Solid Edge part; units mm, degrees
sketch "Sketch1" plane through (0, 0, 0) normal (0, -1, 0) x (1, 0, 0)
  line L0 (270, 170) -> (-270, 170)
  line L1 (-270, 170) -> (-270, -170)
  line L2 (-270, -170) -> (270, -170)
  line L3 (270, -170) -> (270, 170)
  line L4 (330, 230) -> (-330, 230)
  line L5 (-330, 230) -> (-330, -230)
  line L6 (-330, -230) -> (330, -230)
  line L7 (330, -230) -> (330, 230)
extrude "Protrusion1" add sketch "Sketch1" against normal blind 60
sketch "Sketch2" plane through (0, 60, 0) normal (0, 1, 0) x (1, 0, 0)
  line L0 (269.9973, 170.0076) -> (329.9407, 170.0076)
  line L1 (329.9407, 170.0076) -> (329.9407, 229.951)
  line L2 (329.9407, 229.951) -> (269.9973, 229.951)
  line L3 (269.9973, 229.951) -> (269.9973, 170.0076)
extrude "ExtrudedProtrusion_2" add sketch "Sketch2" along normal blind 180
sketch "Sketch3" plane through (329.9407, 150, -199.9793) normal (1, 0, 0) x (0, 0, 1)
  line L0 (-29.9717, -63.4202) -> (29.9717, -63.4202)
  line L1 (29.9717, -63.4202) -> (30.0593, -72.2902)
  line L2 (30.0593, -90.0301) -> (30.0593, -72.2902)
  line L3 (-30.0593, -90.0301) -> (30.0593, -90.0301)
  line L4 (-30.0593, -72.2902) -> (-30.0593, -90.0301)
  line L5 (-30.0593, -72.2902) -> (-29.9717, -63.4202)
extrude "ExtrudedProtrusion_3" add sketch "Sketch3" along normal blind 60
mirror "Mirror1" about plane through (0, 0, 0) normal (-1, 0, 0) of "ExtrudedProtrusion_2", "ExtrudedProtrusion_3"
mirror "Mirror2" about plane through (0, 0, 0) normal (0, 0, 1) of "ExtrudedProtrusion_2", "ExtrudedProtrusion_3"
mirror "Mirror3" about plane through (0, 0, 0) normal (0, 0, 1) of "Mirror1"
sketch "Sketch4" plane through (0, 0, 0) normal (0, -1, 0) x (1, 0, 0)
  circle A0 centre (-300, 152.3787) radius 20
  circle A1 centre (-300, 106.6771) radius 20
  circle A2 centre (-300, 52.3163) radius 20
  circle A3 centre (-300, 0) radius 20
extrude "ExtrudedCutout_8" cut sketch "Sketch4" against normal blind 60
mirror "Mirror4" about plane through (0, 0, 0) normal (-1, 0, 0) of "ExtrudedCutout_8"
mirror "Mirror5" about plane through (0, 0, 0) normal (0, 0, -1) of "ExtrudedCutout_8", "Mirror4"
Input: part model. Units: mm. Frame: model coordinates. A direction names the side the tool comes from. Coordinates: 2 decimals unless noted, no trailing zeros. Write each loop counter-clockwise with the first axis right and the second up, starting at its lowest first coordinate (ties: lowest second). Pieces come first, ordered by that corner, then holes. Notation, with made-up numbers: M 50.5,-9 L 69.5,-9 A21 cw 69.5,-3 Z; hole C -12,17 d6. An arc over 180 degrees is marked long. Use one line per item in the form item = value.
Q1. Material intervals for probe 1 along X at (y, z) = (22, -52); probe 2 along X at (y, z) = (17.5, 22); probe 3 along X at (y, z) = (208.5, -192), sorted ascending. Write a range as from..to.
Answer below:
probe_1 = -330..-320, -280..-270, 270..280, 320..330
probe_2 = -330..-270, 270..330
probe_3 = -329.94..-270, 270..329.94
Q2. Section B-B (z = 0). Return loops of the section in (x, y), plus the area to 3 significant figures.
Answer below:
outline = M -330,0 L -320,0 L -320,60 L -330,60 Z; M -280,0 L -270,0 L -270,60 L -280,60 Z; M 270,0 L 280,0 L 280,60 L 270,60 Z; M 320,0 L 330,0 L 330,60 L 320,60 Z
area = 2,400 mm²
Q3. Section A-A (x = -257). Return loops of the section in (y, z).
Answer below:
outline = M 0,-230 L 60,-230 L 60,-170 L 0,-170 Z; M 0,170 L 60,170 L 60,230 L 0,230 Z
Q4. Set-up query: faces 5 (the face through (360, 231, 169.92)), 6 (the face through (360, 213.42, 200)), 7 (the face through (-360, 213.42, -200)), 8 (the face through (269.997, 149, -200)), 9 (the face through (281.525, 29.58, 7.66)). Return all of +Z, -Z, +X, -X, +Y, -Y with unobstructed straight access to the full face (end or side cutting, diameter ignored); none if empty.
Answer below:
face_5 = +X, -X, +Y, -Y
face_6 = +Z, -Z, +X, -Y
face_7 = +Z, -Z, -X, -Y
face_8 = +Z, -Z, +Y
face_9 = +Y, -Y
Q5. Draft query along Z for faces 1 (the face through (281.525, 29.58, -44.656)), 2 (the face through (-281.525, 29.58, -160.039)), 3 (the face through (360, 231, 230.039)), 4 (the face through (-389.941, 227, -200)). Return one class per face: released by +Z, released by -Z, zero draft, split by the parting line, or undercut.
Answer below:
face_1 = undercut
face_2 = undercut
face_3 = released by +Z
face_4 = zero draft
Q6. First-contact query: pin 1 (18 mm diameter, centred on x = 286, y = 170, fed in from -Z); pin 2 (10 mm diameter, centred on y = 113, z = -169, fed in from -X); pin 3 (1.9 mm diameter, centred on x = -298, z = -171.5, fed in from -Y); pin 4 (1.5 mm diameter, centred on x = 72.5, y = 39.5, fed in from +Z). Flat tips, straight axial feed; report the tip coordinate or a pass-through.
Answer below:
pin_1 = -229.95
pin_2 = -329.94
pin_3 = 0
pin_4 = 230
Q7. Section C-C (y = 34.5). Count the separate pieces of the cut face and the enclosed holes in it, plus the area to 3 significant figures.
Answer below:
separate_pieces = 1
enclosed_holes = 15
area = 102,000 mm²
